```python
from build123d import *

# Parameters (mm, degrees)
SKETCH1_R           = 5
SKETCH1_W           = 10
SKETCH1_H           = 27
BOSS_EXTRUDE1_DEPTH = 60
BOSS_EXTRUDE2_REACH = 89.618
SKETCH2_R           = 4.5
CUT_EXTRUDE1_DEPTH  = 7
BOSS_EXTRUDE3_START = -63
SKETCH4_R           = 9.5
BOSS_EXTRUDE3_DEPTH = 63
BOSS_EXTRUDE5_DEPTH = 50
CUT_EXTRUDE16_DEPTH = 20
CUT_EXTRUDE2_DEPTH  = 3
FILLET1_R           = 7


with BuildPart() as part:
    # Sketch1 → Boss-Extrude1 (new body)
    with BuildSketch(Plane.XY):
        Polygon((-10.392304845, 22.5), (-10.392304845, -22.5), (-5.196152423, -31.5), (5.196152423, -31.5), (10.392304845, -22.5), (10.392304845, 22.5), (5.196152423, 31.5), (-5.196152423, 31.5), align=None)
        with Locations((0, 22.5)):
            Circle(SKETCH1_R, mode=Mode.SUBTRACT)
        with Locations((0, -22.5)):
            Circle(SKETCH1_R, mode=Mode.SUBTRACT)
        Rectangle(SKETCH1_W, SKETCH1_H, mode=Mode.SUBTRACT)
    extrude(amount=BOSS_EXTRUDE1_DEPTH)

    # Boss-Extrude2: up to this face of the body (flat: up to its plane)
    boss_extrude2_end = Plane(part.part.faces().sort_by_distance((0, 13.5, 30))[0])
    # Sketch2 → Boss-Extrude2 (add, up to the picked face)
    with BuildSketch(Plane.XZ.offset(-31.5), mode=Mode.PRIVATE) as boss_extrude2_sk1:
        with BuildLine():
            Line((-30, 25), (-5.196152423, 25))
            Line((-5.196152423, 25), (-5.196152423, 0))
            Line((-5.196152423, 0), (-30, 0))
            ThreePointArc((-30, 0), (-42.5, 12.5), (-30, 25))
        make_face()
        with Locations((-30, 12.5)):
            Circle(SKETCH2_R, mode=Mode.SUBTRACT)
    boss_extrude2_tool1 = split(extrude(boss_extrude2_sk1.sketch, amount=BOSS_EXTRUDE2_REACH, mode=Mode.PRIVATE), bisect_by=boss_extrude2_end, keep=Keep.BOTH, mode=Mode.PRIVATE)
    add(boss_extrude2_tool1.solids().sort_by(Axis((-22.0337, 31.5, 12.5), (0, -1, 0)))[0])

    # Sketch3 → Cut-Extrude1 (cut)
    with BuildSketch(Plane(origin=(0, 13.5, 0), x_dir=(-1, 0, 0), z_dir=(0, -1, 0))):
        Polygon((33.75277675, -6), (26.24722325, -6), (22.494446501, -12.5), (26.24722325, -19), (33.75277675, -19), (37.505553499, -12.5), align=None)
    extrude(amount=-CUT_EXTRUDE1_DEPTH, mode=Mode.SUBTRACT)

    # Sketch4 → Boss-Extrude3 (add)
    with BuildSketch(Plane.XZ.offset(31.5).offset(BOSS_EXTRUDE3_START)):
        with BuildLine():
            Line((-30, 55.5), (-5.196152423, 55.5))
            Line((-5.196152423, 55.5), (-5.196152423, 26.5))
            Line((-5.196152423, 26.5), (-30, 26.5))
            ThreePointArc((-30, 26.5), (-44.5, 41), (-30, 55.5))
        make_face()
        with Locations(Location((-30, 41, 0), (0, 0, 270))):
            Circle(SKETCH4_R, mode=Mode.SUBTRACT)
    extrude(amount=BOSS_EXTRUDE3_DEPTH)

    # Sketch34 → Boss-Extrude5 (add)
    with BuildSketch(Plane.XY.offset(60)):
        with BuildLine():
            Line((-10.392304845, 22.5), (-10.392304845, -22.5))
            Line((-10.392304845, -22.5), (-5, -22.5))
            Line((-5, -22.5), (-5, 22.5))
            ThreePointArc((-5, 22.5), (-3.535533906, 26.035533906), (0, 27.5))
            Line((0, 27.5), (0, 31.5))
            Line((0, 31.5), (-5.196152423, 31.5))
            Line((-5.196152423, 31.5), (-10.392304845, 22.5))
        make_face()
    extrude(amount=BOSS_EXTRUDE5_DEPTH)

    # Sketch26 → Cut-Extrude16 (cut)
    with BuildSketch(Plane(origin=(-5, -6.617020142, 13.078335781), x_dir=(0, 0, -1), z_dir=(1, 0, 0))):
        with BuildLine():
            Line((-89.921664219, 23.867020142), (-86.921664219, 23.867020142))
            ThreePointArc((-86.921664219, 23.867020142), (-85.171664219, 22.117020142), (-86.921664219, 20.367020142))
            Line((-86.921664219, 20.367020142), (-89.921664219, 20.367020142))
            ThreePointArc((-89.921664219, 20.367020142), (-91.671664219, 22.117020142), (-89.921664219, 23.867020142))
        make_face()
        with BuildLine():
            Line((-58.921664219, 23.867020142), (-55.921664219, 23.867020142))
            ThreePointArc((-55.921664219, 23.867020142), (-54.171664219, 22.117020142), (-55.921664219, 20.367020142))
            Line((-55.921664219, 20.367020142), (-58.921664219, 20.367020142))
            ThreePointArc((-58.921664219, 20.367020142), (-60.671664219, 22.117020142), (-58.921664219, 23.867020142))
        make_face()
        with BuildLine():
            Line((-58.921664219, -7.132979858), (-55.921664219, -7.132979858))
            ThreePointArc((-55.921664219, -7.132979858), (-54.171664219, -8.882979858), (-55.921664219, -10.632979858))
            Line((-55.921664219, -10.632979858), (-58.921664219, -10.632979858))
            ThreePointArc((-58.921664219, -10.632979858), (-60.671664219, -8.882979858), (-58.921664219, -7.132979858))
        make_face()
        with BuildLine():
            Line((-89.921664219, -7.132979858), (-86.921664219, -7.132979858))
            ThreePointArc((-86.921664219, -7.132979858), (-85.171664219, -8.882979858), (-86.921664219, -10.632979858))
            Line((-86.921664219, -10.632979858), (-89.921664219, -10.632979858))
            ThreePointArc((-89.921664219, -10.632979858), (-91.671664219, -8.882979858), (-89.921664219, -7.132979858))
        make_face()
        with BuildLine():
            Line((-74.421664219, 14.617020142), (-71.421664219, 14.617020142))
            ThreePointArc((-71.421664219, 14.617020142), (-63.421664219, 6.617020142), (-71.421664219, -1.382979858))
            Line((-71.421664219, -1.382979858), (-74.421664219, -1.382979858))
            ThreePointArc((-74.421664219, -1.382979858), (-82.421664219, 6.617020142), (-74.421664219, 14.617020142))
        make_face()
    extrude(amount=-CUT_EXTRUDE16_DEPTH, mode=Mode.SUBTRACT)

    # Sketch37 → Cut-Extrude2 (cut)
    with BuildSketch(Plane(origin=(-5, 8.494761854, 122.050976771), x_dir=(0, 0, -1), z_dir=(1, 0, 0))):
        with BuildLine():
            Line((22.050976771, 12.255238146), (19.050976771, 12.255238146))
            ThreePointArc((19.050976771, 12.255238146), (13.800976771, 7.005238146), (19.050976771, 1.755238146))
            Line((19.050976771, 1.755238146), (22.050976771, 1.755238146))
            ThreePointArc((22.050976771, 1.755238146), (27.300976771, 7.005238146), (22.050976771, 12.255238146))
        make_face()
        with BuildLine():
            Line((53.050976771, 12.255238146), (50.050976771, 12.255238146))
            ThreePointArc((50.050976771, 12.255238146), (44.800976771, 7.005238146), (50.050976771, 1.755238146))
            Line((50.050976771, 1.755238146), (53.050976771, 1.755238146))
            ThreePointArc((53.050976771, 1.755238146), (58.300976771, 7.005238146), (53.050976771, 12.255238146))
        make_face()
        with BuildLine():
            Line((53.050976771, -18.744761854), (50.050976771, -18.744761854))
            ThreePointArc((50.050976771, -18.744761854), (44.800976771, -23.994761854), (50.050976771, -29.244761854))
            Line((50.050976771, -29.244761854), (53.050976771, -29.244761854))
            ThreePointArc((53.050976771, -29.244761854), (58.300976771, -23.994761854), (53.050976771, -18.744761854))
        make_face()
        with BuildLine():
            Line((19.050976771, -29.244761854), (22.050976771, -29.244761854))
            ThreePointArc((22.050976771, -29.244761854), (27.300976771, -23.994761854), (22.050976771, -18.744761854))
            Line((22.050976771, -18.744761854), (19.050976771, -18.744761854))
            ThreePointArc((19.050976771, -18.744761854), (13.800976771, -23.994761854), (19.050976771, -29.244761854))
        make_face()
    extrude(amount=-CUT_EXTRUDE2_DEPTH, mode=Mode.SUBTRACT)

    # Fillet1
    fillet1_edges = [part.edges().sort_by_distance(p)[0] for p in [
        (-7.696152423, -22.5, 110),
    ]]
    fillet(fillet1_edges, radius=FILLET1_R)


solid = part.part
```
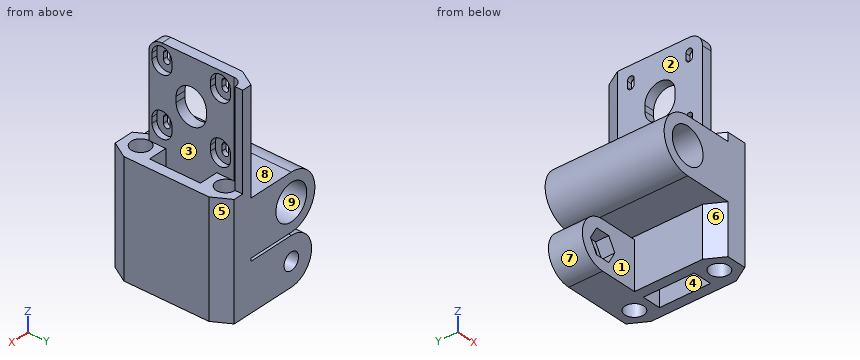
Could you check a few things on this model? Use its own coordinates, in mm. Face numbers are marked on the shaded views. A direction names the side the tool comes from. Round coordinates to 2 decimals unless told otherwise and drop trailing zeros. Loops run counter-clockwise (first coordinate to the right, second up) from the corner with the lowest first, then second, coordinate; pieces in that order, holes last. Notation, with made-up numbers: (40.5, 87.25) -> (92.5, 87.25) arc R18 ccw to (92.5, 99.25) -> close; hole circle Ø6 at (34, 49). An arc over 180 degrees is marked (long way). Put each result on its own line as item: value.
Q1. Please list where these lines run through material, in increasing order: line 1 (X direction, y = 16, z = 41); line 2 (Z direction, x = -33, y = 21.5); line 3 (Y direction, x = 0, z = 32). Write a range as from..to.
Checks:
line 1: -44.5..-39.5, -20.5..10.39
line 2: 0.37..9.15, 15.85..24.63, 26.81..31.99, 50.01..55.19
line 3: -31.5..-27.5, -17.5..-13.5, 13.5..17.5, 27.5..31.5
Q2. I want a section at C-C on y = 1. Write out the boundary of the cut face in (x, z), and give its area (3 significant figures).
Checks:
outline: (-30, 26.5) -> (-10.39, 26.5) -> (-10.39, 0) -> (-5, 0) -> (-5, 76.56) -> (-10.39, 76.56) -> (-10.39, 55.5) -> (-30, 55.5) arc R14.5 ccw to start; (-10.39, 95.44) -> (-5, 95.44) -> (-5, 110) -> (-10.39, 110) -> close; (5, 0) -> (10.39, 0) -> (10.39, 60) -> (5, 60) -> close; hole circle Ø19 at (-30, 41)
area: 1,430 mm2
Q3. Thinking about a two-plate mould opening in Z: for the marked faces 6, 7, 8 and 9, which applies, pulls with the +Z half, pulls with the -Z half, needs draft (parallel to the pull), parting line crosses it, or undercut?
Checks:
face 6: needs draft
face 7: undercut
face 8: pulls with the +Z half
face 9: undercut
Q4. Which directions (+Z, -Z, +X, -X, +Y, -Y) give clear straight access to the entire face, cutting with the end or side of a thin tool? Please do the marked faces 1, 2, 3, 4 and 5.
Checks:
face 1: -Z, -X, -Y
face 2: +Z, -X, +Y, -Y
face 3: +Z
face 4: +Z, -Z
face 5: +Z, -Z, +X, +Y
Q5. I want a section at A-A on z = 101.5. Write out the boundary of the cut face in (x, y), and give its area (3 significant figures).
Checks:
outline: (-10.39, -22.5) -> (-5, -22.5) -> (-5, -20.75) -> (-8, -20.75) -> (-8, -17.25) -> (-10.39, -17.25) -> close; (-10.39, -13.75) -> (-8, -13.75) -> (-8, -10.25) -> (-5, -10.25) -> (-5, 10.25) -> (-8, 10.25) -> (-8, 13.75) -> (-10.39, 13.75) -> close; (-10.39, 17.25) -> (-8, 17.25) -> (-8, 20.75) -> (-5, 20.75) -> (-5, 22.5) arc R5 cw to (0, 27.5) -> (0, 31.5) -> (-5.2, 31.5) -> (-10.39, 22.5) -> close
area: 213 mm2
Q6. I want a section at B-B on x = -15.5. Write out the boundary of the cut face in (y, z), and give its area (3 significant figures).
Checks:
outline: (-31.5, 26.5) -> (31.5, 26.5) -> (31.5, 55.5) -> (-31.5, 55.5) -> close; (13.5, 0) -> (31.5, 0) -> (31.5, 25) -> (13.5, 25) -> close
area: 2,280 mm2
Q7. I want a section at D-D on z = 65.5. Write out the boundary of the cut face in (x, y), and give its area (3 significant figures).
Checks:
outline: (-10.39, -22.5) -> (-5, -22.5) -> (-5, -19.41) -> (-8, -19.41) -> (-8, -11.59) -> (-5, -11.59) -> (-5, 11.59) -> (-8, 11.59) -> (-8, 19.41) -> (-5, 19.41) -> (-5, 22.5) arc R5 cw to (0, 27.5) -> (0, 31.5) -> (-5.2, 31.5) -> (-10.39, 22.5) -> close
area: 246 mm2
Q8. For pin 1 Ø1.2 at (x, z) = (-8.5, 102) entering from -Y; pin 2 Ø0.7 at (x, z) = (-9, 70) entering from +Y; pin 3 Ø1.5 at (x, y) = (-36, -22.5) entering from -Z, each with a flat end and sliding along its axis, tell me the tip position at first contact or that it passes through.
Checks:
pin 1: y = -22.5
pin 2: y = 25.52
pin 3: z = 27.48
